from build123d import *

# Parameters (mm, degrees)
FRONT_PANEL_DEPTH                = 1.905
SKETCH5_R                        = 2.4257
SKETCH5_R_2                      = 2.0701
FRONT_PANEL_MOUNTING_HOLES_DEPTH = 1.905
RACK_MOUNTING_SLOT_DEPTH         = 1.905
ADIO_MOUNTING_HOLES_R            = 1.7399
CUT_EXTRUDE1_DEPTH               = 2.54
SKETCH8_R                        = 6.858
BNC_SEED_HOLE_DEPTH              = 2.54
BNC_PATTERN_COUNT                = 4
BNC_PATTERN_PITCH                = 20.32
BNC_PATTERN_COUNT_DIR2           = 4
BNC_PATTERN_PITCH_DIR2           = 20.32
SKETCH9_W                        = 58.039
SKETCH9_H                        = 10.668
DIO_SEED_HOLE_DEPTH              = 2.54
DIO_PATTERN_COUNT                = 4
DIO_PATTERN_PITCH                = 20.32
LCD_VIEW_CUTOUT_W                = 135.46
LCD_VIEW_CUTOUT_H                = 101.9
LCD_CUTOUT_DEPTH                 = 2.54
LCD_MOUNT_HOLES_R                = 1.5
LCD_MOUNT_HOLE_CUT_DEPTH         = 2.54
SKETCH10_W                       = 12.9
SKETCH10_H                       = 19.2
POWER_SW_CUT_DEPTH               = 12.03
SKETCH11_W                       = 2.935387627
SKETCH11_H                       = 28.1
SKETCH11_W_2                     = 8.128
SKETCH11_H_2                     = 20.828
CUT_EXTRUDE8_DEPTH               = 2.54


# Sheet-metal steps are written as plain solids
with BuildPart() as part:
    # Sketch1 → Front Panel (new body)
    with BuildSketch(Plane.XY):
        with BuildLine():
            Line((1.016, 0), (481.584, 0))
            ThreePointArc((481.584, 0), (482.30242049, 0.29757951), (482.6, 1.016))
            Line((482.6, 1.016), (482.6, 131.572))
            ThreePointArc((482.6, 131.572), (482.30242049, 132.29042049), (481.584, 132.588))
            Line((481.584, 132.588), (1.016, 132.588))
            ThreePointArc((1.016, 132.588), (0.29757951, 132.29042049), (0, 131.572))
            Line((0, 131.572), (0, 1.016))
            ThreePointArc((0, 1.016), (0.29757951, 0.29757951), (1.016, 0))
        make_face()
    extrude(amount=FRONT_PANEL_DEPTH)

    # Sketch5 → Front Panel Mounting Holes (cut)
    with BuildSketch(Plane.XY.offset(1.905)):
        with Locations((445.135, 21.844)):
            Circle(SKETCH5_R)
        with Locations((37.465, 21.844)):
            Circle(SKETCH5_R)
        with Locations((37.465, 110.744)):
            Circle(SKETCH5_R)
        with Locations((445.135, 110.744)):
            Circle(SKETCH5_R)
        with Locations((241.3, -19.907000064)):
            Circle(SKETCH5_R_2)
    extrude(amount=-FRONT_PANEL_MOUNTING_HOLES_DEPTH, mode=Mode.SUBTRACT)

    # Sketch2 → Rack Mounting Slot (cut)
    with BuildSketch(Plane.XY.offset(1.905)):
        with BuildLine():
            Line((472.7575, 34.1503), (475.9579, 34.1503))
            ThreePointArc((475.9579, 34.1503), (479.5012, 37.6936), (475.9579, 41.2369))
            Line((475.9579, 41.2369), (472.7575, 41.2369))
            ThreePointArc((472.7575, 41.2369), (469.2142, 37.6936), (472.7575, 34.1503))
        make_face()
        with BuildLine():
            Line((9.8425, 98.4377), (6.6421, 98.4377))
            ThreePointArc((6.6421, 98.4377), (3.0988, 94.8944), (6.6421, 91.3511))
            Line((6.6421, 91.3511), (9.8425, 91.3511))
            ThreePointArc((9.8425, 91.3511), (13.3858, 94.8944), (9.8425, 98.4377))
        make_face()
        with BuildLine():
            Line((6.6421, 41.2369), (9.8425, 41.2369))
            ThreePointArc((9.8425, 41.2369), (13.3858, 37.6936), (9.8425, 34.1503))
            Line((9.8425, 34.1503), (6.6421, 34.1503))
            ThreePointArc((6.6421, 34.1503), (3.0988, 37.6936), (6.6421, 41.2369))
        make_face()
        with BuildLine():
            Line((475.9579, 91.3511), (472.7575, 91.3511))
            ThreePointArc((472.7575, 91.3511), (469.2142, 94.8944), (472.7575, 98.4377))
            Line((472.7575, 98.4377), (475.9579, 98.4377))
            ThreePointArc((475.9579, 98.4377), (479.5012, 94.8944), (475.9579, 91.3511))
        make_face()
    extrude(amount=-RACK_MOUNTING_SLOT_DEPTH, mode=Mode.SUBTRACT)

    # ADio mounting holes → Cut-Extrude1 (cut)
    with BuildSketch(Plane.XY.offset(1.905)):
        with Locations((49.53, 121.158)):
            Circle(ADIO_MOUNTING_HOLES_R)
        with Locations((113.03, 121.158)):
            Circle(ADIO_MOUNTING_HOLES_R)
        with Locations((232.41, 121.158)):
            Circle(ADIO_MOUNTING_HOLES_R)
        with Locations((49.53, 24.638)):
            Circle(ADIO_MOUNTING_HOLES_R)
        with Locations((113.03, 24.638)):
            Circle(ADIO_MOUNTING_HOLES_R)
        with Locations((232.41, 24.638)):
            Circle(ADIO_MOUNTING_HOLES_R)
    extrude(amount=-CUT_EXTRUDE1_DEPTH, mode=Mode.SUBTRACT)

    # Sketch8 → BNC seed hole (cut)
    with BuildSketch(Plane.XY.offset(1.905)):
        with Locations((64.77, 105.918)):
            Circle(SKETCH8_R)
    bnc_seed_hole = extrude(amount=-BNC_SEED_HOLE_DEPTH, mode=Mode.SUBTRACT)

    # BNC pattern: BNC seed hole 4 × 4
    with Locations(*[(i * BNC_PATTERN_PITCH, -j * BNC_PATTERN_PITCH_DIR2, 0) for i in range(BNC_PATTERN_COUNT) for j in range(BNC_PATTERN_COUNT_DIR2) if (i, j) != (0, 0)]):
        add(bnc_seed_hole, mode=Mode.SUBTRACT)

    # Sketch9 → DIO Seed Hole (cut)
    with BuildSketch(Plane.XY.offset(1.905)):
        with Locations((212.4075, 105.918)):
            Rectangle(SKETCH9_W, SKETCH9_H)
    dio_seed_hole = extrude(amount=-DIO_SEED_HOLE_DEPTH, mode=Mode.SUBTRACT)

    # DIO Pattern: DIO Seed Hole ×4
    with Locations(*[(0, -i * DIO_PATTERN_PITCH, 0) for i in range(1, DIO_PATTERN_COUNT)]):
        add(dio_seed_hole, mode=Mode.SUBTRACT)

    # LCD view cutout → LCD Cutout (cut)
    with BuildSketch(Plane.XY.offset(1.905)):
        with Locations((335.534, 66.294)):
            Rectangle(LCD_VIEW_CUTOUT_W, LCD_VIEW_CUTOUT_H)
    extrude(amount=-LCD_CUTOUT_DEPTH, mode=Mode.SUBTRACT)

    # LCD mount holes → LCD mount hole - cut (cut)
    with BuildSketch(Plane.XY.offset(1.905)):
        with Locations((259.03, 112.498)):
            Circle(LCD_MOUNT_HOLES_R)
        with Locations((411.53, 112.498)):
            Circle(LCD_MOUNT_HOLES_R)
        with Locations((259.03, 20.598)):
            Circle(LCD_MOUNT_HOLES_R)
        with Locations((411.53, 20.598)):
            Circle(LCD_MOUNT_HOLES_R)
    extrude(amount=-LCD_MOUNT_HOLE_CUT_DEPTH, mode=Mode.SUBTRACT)

    # Sketch10 → power sw - cut (cut)
    with BuildSketch(Plane.XY.offset(1.905)):
        with Locations((428.525, 110.288)):
            Rectangle(SKETCH10_W, SKETCH10_H)
    extrude(amount=-POWER_SW_CUT_DEPTH, mode=Mode.SUBTRACT)

    # Sketch11 → Cut-Extrude8 (cut)
    with BuildSketch(Plane.XY.offset(1.905)):
        with Locations((428.512093814, 73.405799856)):
            Rectangle(SKETCH11_W, SKETCH11_H)
        with Locations((427.6344, 36.825799856)):
            Rectangle(SKETCH11_W_2, SKETCH11_H_2)
    extrude(amount=-CUT_EXTRUDE8_DEPTH, mode=Mode.SUBTRACT)


solid = part.part
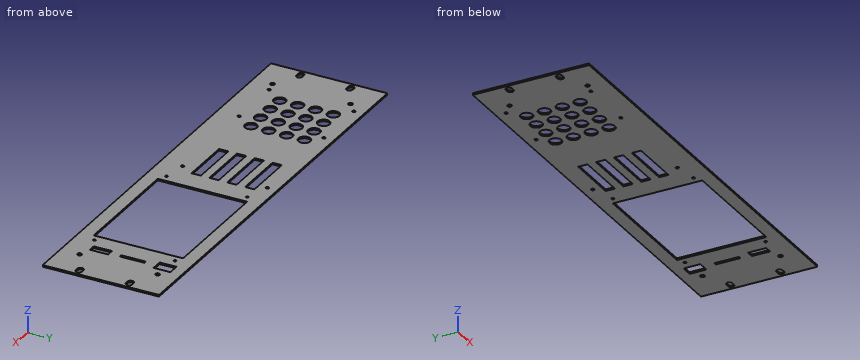
Source: CAD feature listing. Evaluate the final solid. Frame: model axes, mm. Coordinates: 2 decimals unless noted, no trailing zeros. Loops run counter-clockwise (first coordinate to the right, second up) from the corner with the lowest first, then second, coordinate; pieces in that order, holes last. Notation, with made-up numbers: (39.25, 12.25) - (45.25, 12.25) arc R32 ccw to (45.25, 50.25) - close; hole circle Ø2 at (-39.5, -35). An arc over 180 degrees is marked (long way). Return JSON: item names as keys, results as strings.
Q1. Contact query for a flat-ended pin moving along its axis: P1, Ø12.5, axis at x = 125.73, y = 65.278, coming from the -Z side. Output: stop coordinate, or through.
Results:
{"P1": "through"}
Q2. Section A-A, the plane x = 85.09. Return loops of the section in (y, z) (3 decimals).
Results:
{"outline": "(0, 0) - (38.1, 0) - (38.1, 1.905) - (0, 1.905) - close; (51.816, 0) - (58.42, 0) - (58.42, 1.905) - (51.816, 1.905) - close; (72.136, 0) - (78.74, 0) - (78.74, 1.905) - (72.136, 1.905) - close; (92.456, 0) - (99.06, 0) - (99.06, 1.905) - (92.456, 1.905) - close; (112.776, 0) - (132.588, 0) - (132.588, 1.905) - (112.776, 1.905) - close"}
Q3. Section B-B, the plane z = 1.2. Give the number of separate pieces and of enclosed holes in the cut face, plus the area to 3 significant figures.
Results:
{"separate pieces": "1", "enclosed holes": "42", "area": "44,400 mm2"}
Q4. Material intervals for line 1 along X through (y, z) = (38, 1); line 2 along Y through (x, z) = (215, 0.9); line 3 along Y through (x, z) = (125.73, 0.65), sorted ascending.
Results:
{"line 1": "0 to 3.11, 13.37 to 267.8, 403.26 to 423.57, 431.7 to 469.23, 479.49 to 482.6", "line 2": "0 to 39.62, 50.29 to 59.94, 70.61 to 80.26, 90.93 to 100.58, 111.25 to 132.59", "line 3": "0 to 38.1, 51.82 to 58.42, 72.14 to 78.74, 92.46 to 99.06, 112.78 to 132.59"}
